```python
from build123d import *

# Parameters (mm, degrees)
SKETCH_1_W          = 12
SKETCH_1_H          = 14
SKETCH_1_R          = 1.75
EXTRUDE_1_DEPTH     = 5
SKETCH_2_W          = 16.082841594
SKETCH_2_H          = 10
CUT_EXTRUDE_1_DEPTH = 2


with BuildPart() as part:
    # Эскиз1 → Вытянуть1 (new body)
    with BuildSketch(Plane.XY):
        Rectangle(SKETCH_1_W, SKETCH_1_H)
        with Locations((0, -3.5)):
            Circle(SKETCH_1_R, mode=Mode.SUBTRACT)
    extrude(amount=EXTRUDE_1_DEPTH)

    # Эскиз2 → Вырез-Вытянуть1 (cut)
    with BuildSketch(Plane.XY.offset(5)):
        with Locations((-0.230919178, 4)):
            Rectangle(SKETCH_2_W, SKETCH_2_H)
    extrude(amount=-CUT_EXTRUDE_1_DEPTH, mode=Mode.SUBTRACT)


solid = part.part
```
Verification items for the finished model (mm, model axes). A direction names the side the tool comes from. Coordinates: 2 decimals unless noted, no trailing zeros. Order: outer loops, then holes, each group sorted by start corner. A loop starts at its lowest first (then second) coordinate and runs counter-clockwise, first axis right, second up. Notation, with made-up numbers: (25, -1.5) - (82, -1.5) arc R25 cw to (82, 33.5) - close; hole circle Ø3 at (-32.5, 64). An arc over 180 degrees is marked (long way). Return JSON: item names as keys, results as strings.
(1) Section check B-B, the plane y = -3.5. Record the cut outline in (x, z), and give its area (3 significant figures).
Filled sheet:
{"outline": "(-6, 0) - (-1.75, 0) - (-1.75, 5) - (-6, 5) - close; (1.75, 0) - (6, 0) - (6, 5) - (1.75, 5) - close", "area": "42.5 mm^2"}
(2) Section check C-C, the plane x = 4.5. Record the cut outline in (y, z).
Filled sheet:
{"outline": "(-7, 0) - (7, 0) - (7, 3) - (-1, 3) - (-1, 5) - (-7, 5) - close"}
(3) Go/stop test with a flat-tipped pin: pin 1 (2.5 mm diameter, centred on x = 2, y = 4.5, fed in from +Z). Record where the tip stops, or that it passes through.
Filled sheet:
{"pin 1": "stops at z = 3"}
(4) Access from +Z, -Z, +X, -X, +Y, -Y to the whole of each face (thin tool, end or side, straight path). Record for faces 1 (the flat face through (0, -1, 4)), 2 (the flat face through (6, -2, 2)).
Filled sheet:
{"face 1": "+Z, +X, -X, +Y", "face 2": "+Z, -Z, +X, +Y, -Y"}
(5) Section check D-D, the plane z = 1.9. Record the cut outline in (x, y), and give its area (3 significant figures).
Filled sheet:
{"outline": "(-6, -7) - (6, -7) - (6, 7) - (-6, 7) - close; hole circle Ø3.5 at (0, -3.5)", "area": "158 mm^2"}
(6) Section check A-A, the plane x = 0. Record the cut outline in (y, z), and give its area (3 significant figures).
Filled sheet:
{"outline": "(-7, 0) - (-5.25, 0) - (-5.25, 5) - (-7, 5) - close; (-1.75, 0) - (7, 0) - (7, 3) - (-1, 3) - (-1, 5) - (-1.75, 5) - close", "area": "36.5 mm^2"}
(7) Thickness scan on line 1 along Y through (x, z) = (0, 1.05); line 2 along Y through (x, z) = (0, 3.45); line 3 along Z through (x, y) = (5.25, 1). Record the ranges inside material, lowest first.
Filled sheet:
{"line 1": "y = -7 to -5.25, -1.75 to 7", "line 2": "y = -7 to -5.25, -1.75 to -1", "line 3": "z = 0 to 3"}
(8) Mould release check, pull along X, two halves, no side actions. Record for faces 3 (the cylindrical face through (-0.38, -5.21, 2.46)), 4 (the flat face through (-6, -2, 2)), 5 (the flat face through (0, 3, 3)): pulls with the +X half, pulls with the -X half, needs draft (parallel to the pull), parting line crosses it, or undercut.
Filled sheet:
{"face 3": "undercut", "face 4": "pulls with the -X half", "face 5": "needs draft"}
